Source: CAD feature listing. Evaluate the final solid. Frame: model axes, mm. A direction names the side the tool comes from. Give positions to 0.01 mm unless a question says otherwise; leave off trailing zeros. Write each loop counter-clockwise with the first axis right and the second up, starting at its lowest first coordinate (ties: lowest second). Pieces come first, ordered by that corner, then holes.
```python
from build123d import *

# Parameters (mm, degrees)
F0_W      = 101.6
F0_H      = 101.6
F1_DEPTH  = 101.6
F3_R      = 38.1
F4_DEPTH  = 184.15
F5_R      = 6.35
F6_DEPTH  = 12.7
F7_R      = 9.525
F8_DEPTH  = 25.4
F9_R      = 12.7
F9_R_2    = 9.525
F10_DEPTH = 25.4


with BuildPart() as f1:
    # F0 (on Right) → F1 (new body, symmetric)
    with BuildSketch(Plane.YZ):
        Rectangle(F0_W, F0_H)
    extrude(amount=F1_DEPTH, both=True)

    # F3 (on offset) → F4 (cut)
    with BuildSketch(Plane.YZ.offset(88.9)):
        Circle(F3_R)
    extrude(amount=-F4_DEPTH, mode=Mode.SUBTRACT)

    # F5 (on face) → F6 (cut, through all)
    with BuildSketch(Plane.YZ.offset(101.6)):
        Circle(F5_R)
    extrude(amount=-F6_DEPTH, mode=Mode.SUBTRACT)

    # F7 (on face) → F8 (cut)
    with BuildSketch(Plane.XY.offset(50.8)):
        with Locations((-82.55, 0)):
            Circle(F7_R)
        with Locations((76.2, 0)):
            Circle(F7_R)
    extrude(amount=-F8_DEPTH, mode=Mode.SUBTRACT)

    # F9 (on face) → F10 (join)
    with BuildSketch(Plane.XY.offset(50.8)):
        with Locations((-82.55, 0)):
            Circle(F9_R)
        with Locations((-82.55, 0)):
            Circle(F9_R_2, mode=Mode.SUBTRACT)
        with Locations((76.2, 0)):
            Circle(F9_R)
        with Locations((76.2, 0)):
            Circle(F9_R_2, mode=Mode.SUBTRACT)
    extrude(amount=F10_DEPTH)


solid = f1.part
```
1. Access query for faces 1 (the cylindrical face through (95.34, -1.38, -6.2)), 2 (the cylindrical face through (63.512, 0.558, 63.322)), 3 (the flat face through (88.9, 8, 1)). Directions: +Z, -Z, +X, -X, +Y, -Y. A direction counts if a zero-diameter tool reaches every point of the face in a straight line with its end or side. Return the directions, or none.
2. Contact query for flat-ended pins moving along their axis: P1, Ø15, axis at x = 76.2, y = 0, coming from the +Z side; P2, Ø12, axis at x = 54.5, y = 14, coming from the +Z side. Output: stop coordinate, or through.
3. Cut plane B-B, the plane x = -49. Return the cut outline in (y, z).
4. Cut plane D-D, the plane x = -82.55. Return the cut outline in (y, z) (3 decimals).
5. Line query: L1, parallel to Z at x = -30, y = 0; L2, parallel to X at y = 6.5, z = -35; L3, parallel to X at y = 0, z = 46 (3 decimals). Output: solid intervals per line, ascending.
6. Cut plane A-A, the plane y = 0. Return the cut outline in (x, z) (3 decimals), then the cut area to 3 significant figures.
7. Cut plane C-C, the plane z = 21. Return the cut outline in (x, y), then the cut area to 3 significant figures.
8. Mould query, pull axis X, two halves, no side actions, for faces 4 (the cylindrical face through (-95.238, 0.558, 63.322)), 5 (the flat face through (101.6, 11, 1)), 6 (the flat face through (-95.25, -1, 1)), 7 (the flat face through (-80.7, 9.5, 76.2)). Classes: +X half, -X half, draft (parallel to the pull), parting line (faces both ways), or undercut.
Response values:
1. face 1: +X
1. face 2: +Z
1. face 3: none
2. P1: stops at z = -37.35
2. P2: stops at z = 50.8
3. outline: (-50.8, -50.8) - (50.8, -50.8) - (50.8, 50.8) - (-50.8, 50.8) - close; hole circle Ø76.2 at (0, 0)
4. outline: (-50.8, -50.8) - (50.8, -50.8) - (50.8, 50.8) - (12.7, 50.8) - (12.7, 76.2) - (9.525, 76.2) - (9.525, 36.89) arc R38.1 cw (long way) to (-9.525, 36.89) - (-9.525, 76.2) - (-12.7, 76.2) - (-12.7, 50.8) - (-50.8, 50.8) - close
5. L1: z = -50.8 to -38.1, 38.1 to 50.8
5. L2: x = -101.6 to -95.25, 88.9 to 101.6
5. L3: x = -101.6 to -92.075, -73.025 to 66.675, 85.725 to 101.6
6. outline: (-101.6, -50.8) - (101.6, -50.8) - (101.6, -6.35) - (88.9, -6.35) - (88.9, -38.1) - (-95.25, -38.1) - (-95.25, 38.1) - (-92.075, 38.1) - (-92.075, 76.2) - (-95.25, 76.2) - (-95.25, 50.8) - (-101.6, 50.8) - close; (-73.025, 38.1) - (66.675, 38.1) - (66.675, 76.2) - (63.5, 76.2) - (63.5, 50.8) - (-69.85, 50.8) - (-69.85, 76.2) - (-73.025, 76.2) - close; (85.725, 38.1) - (88.9, 38.1) - (88.9, 6.35) - (101.6, 6.35) - (101.6, 50.8) - (88.9, 50.8) - (88.9, 76.2) - (85.725, 76.2) - close
6. area: 6,290 mm2
7. outline: (-101.6, -50.8) - (101.6, -50.8) - (101.6, 50.8) - (-101.6, 50.8) - close; hole (-95.25, -31.79) - (88.9, -31.79) - (88.9, 31.79) - (-95.25, 31.79) - close
7. area: 8,940 mm2
8. face 4: undercut
8. face 5: +X half
8. face 6: undercut
8. face 7: draft
